Source: CAD feature listing. Evaluate the final solid. Frame: model axes, mm. Coordinates: 2 decimals unless noted, no trailing zeros. Write each loop counter-clockwise with the first axis right and the second up, starting at its lowest first coordinate (ties: lowest second). Pieces come first, ordered by that corner, then holes. Notation, with made-up numbers: (4, 36) - (43, 36) arc R22 ccw to (43, 70) - close; hole circle Ø2 at (46.5, 83.25). An arc over 180 degrees is marked (long way). One line per item, written item: value.
from build123d import *

# Parameters (mm, degrees)
SKETCH1_R                        = 2.5796875
BOSS_EXTRUDE1_DEPTH              = 3.175
F_10_32_TAPPED_HOLE3_D           = 4.0386
F_10_32_TAPPED_HOLE3_CSINK_D     = 6.096
F_10_32_TAPPED_HOLE3_CSINK_ANGLE = 90


with BuildPart() as part:
    # Sketch1 → Boss-Extrude1 (new body)
    with BuildSketch(Plane(origin=(0, 0, 0), x_dir=(1, 0, 0), z_dir=(0, 1, 0))):
        with BuildLine():
            Line((-47.625, 6.35), (47.625, 6.35))
            ThreePointArc((47.625, 6.35), (53.975, 0), (47.625, -6.35))
            Line((47.625, -6.35), (-47.625, -6.35))
            ThreePointArc((-47.625, -6.35), (-53.975, 0), (-47.625, 6.35))
        make_face()
        with Locations((47.625, 0)):
            Circle(SKETCH1_R, mode=Mode.SUBTRACT)
        with Locations((-47.625, 0)):
            Circle(SKETCH1_R, mode=Mode.SUBTRACT)
    extrude(amount=BOSS_EXTRUDE1_DEPTH)

    # #10-32 Tapped Hole3 (through all)
    with Locations(Plane(origin=(0, 3.175, 0), x_dir=(1, 0, 0), z_dir=(0, 1, 0))):
        with Locations((-47.625, 0), (47.625, 0)):
            CounterSinkHole(F_10_32_TAPPED_HOLE3_D / 2, F_10_32_TAPPED_HOLE3_CSINK_D / 2, counter_sink_angle=F_10_32_TAPPED_HOLE3_CSINK_ANGLE)


solid = part.part
1) Section query C-C on z = 4.25. Output: boundary loops of the cut face in (x, y) (3 decimals), then the cut area to 3 significant figures.
Values found:
outline: (-52.343, 0) - (52.343, 0) - (52.343, 3.175) - (-52.343, 3.175) - close
area: 332 mm2
2) Section query A-A on z = 0. Output: boundary loops of the cut face in (x, y) (3 decimals).
Values found:
outline: (-53.975, 0) - (-50.205, 0) - (-50.205, 2.707) - (-50.673, 3.175) - (-53.975, 3.175) - close; (-45.045, 0) - (45.045, 0) - (45.045, 2.707) - (44.577, 3.175) - (-44.577, 3.175) - (-45.045, 2.707) - close; (50.205, 0) - (53.975, 0) - (53.975, 3.175) - (50.673, 3.175) - (50.205, 2.707) - close
3) Material intervals for line 1 (X direction, y = 0.85, z = 0) (3 decimals); line 2 (X direction, y = 0.7, z = -2); line 3 (X direction, y = 1.85, z = 4.75), sorted ascending.
Values found:
line 1: -53.975 to -50.205, -45.045 to 45.045, 50.205 to 53.975
line 2: -53.65 to -49.25, -46 to 46, 49.25 to 53.65
line 3: -51.84 to 51.84
4) Section query B-B on y = 0.55. Output: boundary loops of the cut face in (x, z) (3 decimals).
Values found:
outline: (-47.625, -6.35) - (47.625, -6.35) arc R6.35 ccw to (47.625, 6.35) - (-47.625, 6.35) arc R6.35 ccw to start; hole circle Ø5.159 at (-47.625, 0); hole circle Ø5.159 at (47.625, 0)
5) Draft query along Z for faces 1 (the cylindrical face through (-45.242, 1.334, 0.988)), 2 (the flat face through (1, 3.175, 0)), 3 (the cylindrical face through (-53.973, 1.565, 0.14)). Return one class per face: released by +Z, released by -Z, zero draft, split by the parting line, or undercut.
Values found:
face 1: undercut
face 2: zero draft
face 3: split by the parting line
